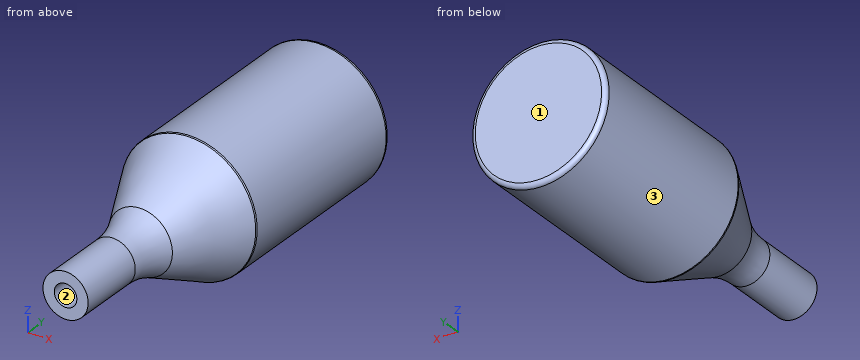
from build123d import *

# Parameters (mm, degrees)
SKETCH1_R          = 30.591778674
CUT_EXTRUDE1_DEPTH = 34
FILLET1_R          = 2


with BuildPart() as part:
    # Esquisse1 → Révolution1 (revolve)
    with BuildSketch(Plane.XY, mode=Mode.PRIVATE) as r_volution1_sk:
        with BuildLine():
            Line((0, 0), (28, 0))
            ThreePointArc((28, 0), (29.414213562, -0.585786438), (30, -2))
            Line((30, -2), (30, -119.627445758))
            ThreePointArc((30, -119.627445758), (29.957782489, -119.990033798), (29.833388678, -120.333222644))
            Line((29.833388678, -120.333222644), (14.22291236, -151.55417528))
            ThreePointArc((14.22291236, -151.55417528), (11.070040421, -160.252602278), (10, -169.4427191))
            Line((10, -169.4427191), (10, -200))
            Line((10, -200), (5, -200))
            Line((5, -200), (5, -170))
            Line((5, -170), (0, -170))
            Line((0, -170), (0, 0))
        make_face()
    revolve(r_volution1_sk.sketch.rotate(Axis((0, 0, 0), (0, -1, 0)), 180), axis=Axis((0, 0, 0), (0, -1, 0)))

    # Sketch1 → Cut-Extrude1 (cut)
    with BuildSketch(Plane(origin=(0, 0, 0), x_dir=(1, 0, 0), z_dir=(0, 1, 0))):
        Circle(SKETCH1_R)
    extrude(amount=-CUT_EXTRUDE1_DEPTH, mode=Mode.SUBTRACT)

    # Fillet1
    fillet1_edges = [part.edges().sort_by_distance(p)[0] for p in [
        (30, -34, 0),
    ]]
    fillet(fillet1_edges, radius=FILLET1_R)


solid = part.part
Input: part model. Units: mm. Frame: model coordinates. Face numbers are marked on the shaded views. Round coordinates to 2 decimals unless told otherwise and drop trailing zeros. Order: outer loops, then holes, each group sorted by start corner. A loop starts at its lowest first (then second) coordinate and runs counter-clockwise, first axis right, second up. Notation, with made-up numbers: (-35.5, -32.5) - (-8.5, -32.5) arc R15 cw to (-8.5, -4.5) - close; hole circle Ø3 at (87.5, -12.5). An arc over 180 degrees is marked (long way). Answer as a JSON object with one key per item and string values. Group by question number.
(1) Cut plane A-A (z = 0). Return loops of the section in (x, y), then the cut area to 3 significant figures.
(2) Cut plane C-C (y = -141). Return loops of the section in (x, z), then the cut area to 3 significant figures.
(3) Pin query (flat end, axial travel): P1, Ø5, axis at x = 2, z = -1, coming from the -Y side; P2, Ø3, axis at y = -97, z = 16, coming from the +X side; P3, Ø2, axis at y = -172, z = 3, coming from the -X side. Return the tip coordinate at first contact, or that it passes through.
(4) Material intervals for probe 1 along Z at (x, y) = (0, -180.25); probe 2 along Y at (x, z) = (2, 18); probe 3 along Y at (x, z) = (25, 13.5), sorted ascending. Write a range as from..to.
(5) Cut plane B-B (x = 0). Return loops of the section in (y, z), then the cut area to 3 significant figures.
(6) Cut plane D-D (y = -46.5). Return loops of the section in (x, z).
(7) Draft query along Z for the marked faces 1, 2 and 3. Return one class per face: released by +Z, released by -Z, zero draft, split by the parting line, or undercut.
Here are the results:
{
 "1": {"outline": "(-30, -119.63) arc R1.58 ccw to (-29.83, -120.33) - (-14.22, -151.55) arc R40 cw to (-10, -169.44) - (-10, -200) - (-5, -200) - (-5, -170) - (5, -170) - (5, -200) - (10, -200) - (10, -169.44) arc R40 cw to (14.22, -151.55) - (29.83, -120.33) arc R1.58 ccw to (30, -119.63) - (30, -36) arc R2 ccw to (28, -34) - (-28, -34) arc R2 ccw to (-30, -36) - close", "area": "7,270 mm^2"},
 "2": {"outline": "circle Ø39 at (0, 0)", "area": "1,190 mm^2"},
 "3": {"P1": "stops at y = -170", "P2": "stops at x = 26.26", "P3": "stops at x = -9.8"},
 "4": {"probe 1": "z = -10..-5, 5..10", "probe 2": "y = -143.78..-34", "probe 3": "y = -123.18..-34.04"},
 "5": {"outline": "(-200, -10) - (-169.44, -10) arc R40 cw to (-151.55, -14.22) - (-120.33, -29.83) arc R1.58 ccw to (-119.63, -30) - (-36, -30) arc R2 ccw to (-34, -28) - (-34, 28) arc R2 ccw to (-36, 30) - (-119.63, 30) arc R1.58 ccw to (-120.33, 29.83) - (-151.55, 14.22) arc R40 cw to (-169.44, 10) - (-200, 10) - (-200, 5) - (-170, 5) - (-170, -5) - (-200, -5) - close", "area": "7,270 mm^2"},
 "6": {"outline": "circle Ø60 at (0, 0)"},
 "7": {"face 1": "zero draft", "face 2": "undercut", "face 3": "split by the parting line"}
}
